For this review, use the dimensioned drawing (mm, ordinates from the lowest corner) and the shaded views. Give positions to 0.01 mm unless a question says otherwise; leave off trailing zeros. Order: outer loops, then holes, each group sorted by start corner. A loop starts at its lowest first (then second) coordinate and runs counter-clockwise, first axis right, second up. Notation, with made-up numbers: (-31, 50.5) -> (28, 50.5) arc R21 cw to (28, 61.5) -> close; hole circle Ø1 at (73, 12.25). An arc over 180 degrees is marked (long way). Return JSON: item names as keys, results as strings.
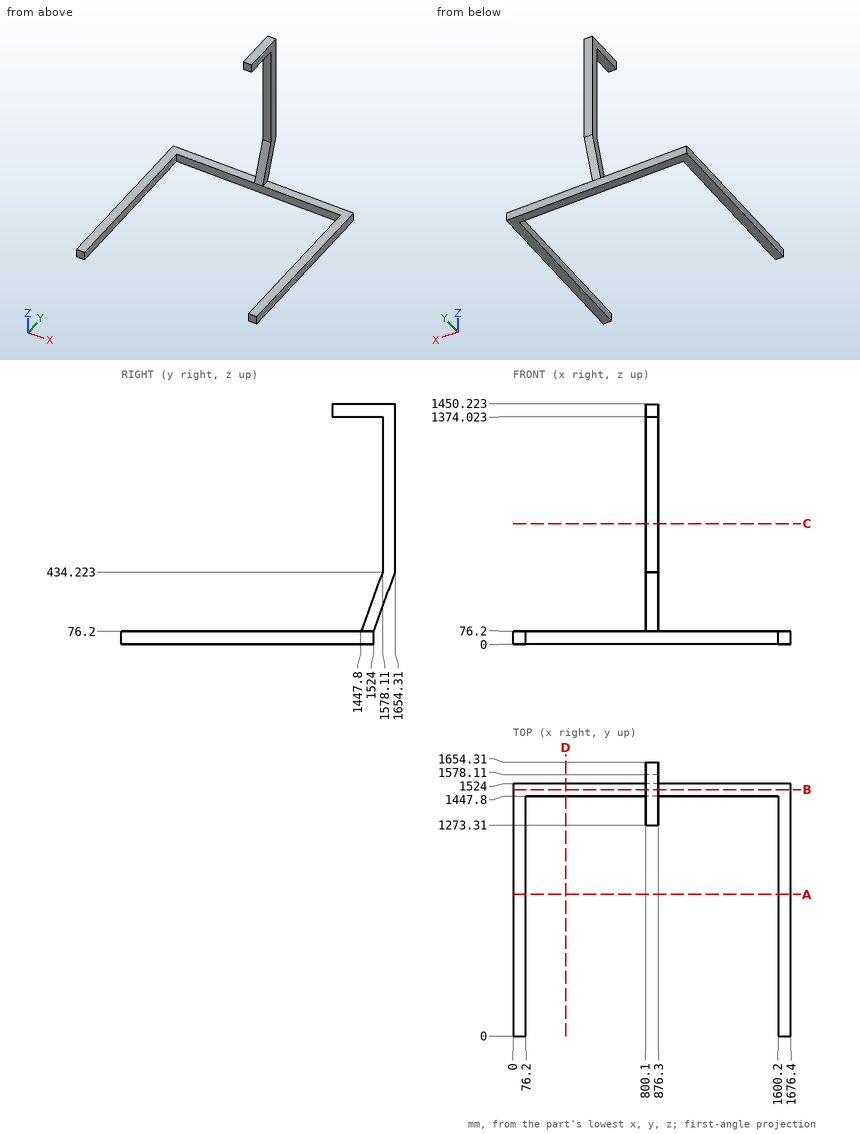
Item 1: Add section A-A (y = 855). Give the boundary of the cut face in (x, z).
Result set:
{"outline": "(0, 0) -> (76.2, 0) -> (76.2, 76.2) -> (0, 76.2) -> close; (1600.2, 0) -> (1676.4, 0) -> (1676.4, 76.2) -> (1600.2, 76.2) -> close"}
Item 2: Add section D-D (x = 317.5). Give the boundary of the cut face in (y, z), plus the area to 3 significant figures.
Result set:
{"outline": "(1447.8, 0) -> (1524, 0) -> (1524, 76.2) -> (1447.8, 76.2) -> close", "area": "5,810 mm^2"}
Item 3: Add section C-C (z = 727.5). Give the boundary of the cut face in (x, y), plus the area to 3 significant figures.
Result set:
{"outline": "(800.1, 1578.11) -> (876.3, 1578.11) -> (876.3, 1654.31) -> (800.1, 1654.31) -> close", "area": "5,810 mm^2"}
Item 4: For pin 1 (23 mm diameter, centred on x = 840.5, z = 1396, fed in from -Y); pin 2 (23 mm diameter, centred on x = 1180.5, z = 34, fed in from -Y), all flat-tipped, find the tip position at first contact; note any pin that passes through.
Result set:
{"pin 1": "stops at y = 1273.31", "pin 2": "stops at y = 1447.8"}
Item 5: Add section B-B (y = 1488). Give the boundary of the cut face in (x, z), plus the area to 3 significant figures.
Result set:
{"outline": "(0, 0) -> (1676.4, 0) -> (1676.4, 76.2) -> (876.3, 76.2) -> (876.3, 186.65) -> (800.1, 186.65) -> (800.1, 76.2) -> (0, 76.2) -> close; (800.1, 1374.02) -> (876.3, 1374.02) -> (876.3, 1450.22) -> (800.1, 1450.22) -> close", "area": "142,000 mm^2"}
Item 6: Wall thickness on L1, parallel to Z at x = 1609.5, y = 1046: over which ranges is the line inside the solid? List them lowest first. Write a range as [from, to].
Result set:
{"L1": "z = [0, 76.2]"}
